Build history of the part. All positions in model axes, mm. Give positions to 0.01 mm unless a question says otherwise; leave off trailing zeros. Loops run counter-clockwise (first coordinate to the right, second up) from the corner with the lowest first, then second, coordinate; pieces in that order, holes last. Notation, with made-up numbers: (-39, 13) -> (12, 13) arc R17 cw to (12, 41) -> close; hole circle Ø2 at (-29.75, -23.75). An arc over 180 degrees is marked (long way). One line per question, with ' | ' between items. Start each with the question number.
(1) Slice it at B-B, the plane y = 7.5. Write the cut outline in (x, z).
(2) Mould opens along X. For faces 1 (the face through (2.37, 8.49, -2.08)), 2 (the face through (0, 8, -49)), 3 (the face through (3, 13, -1)) say: pulls with the +X half, pulls with the -X half, needs draft (parallel to the pull), parting line crosses it, or undercut.
(3) Slice it at A-A, the plane z = -6.4. Write the cut outline in (x, y), then the cut area to 3 significant figures.
(4) Slice it at C-C, the plane x = 2.5. Write the cut outline in (y, z).
(5) Flat gauge pins, fed straight in: pin 1 Ø1 at (x, y) = (0.5, 11.5) entering from +Z; pin 2 Ø1.5 at (x, y) = (4.5, 3.5) entering from -Z. Where does each tip first touch, or does it go through?
(6) Drill centre lines: L1, parallel to X at y = 7.5, z = -1.4; L2, parallel to Y at x = 2.75, z = -6.4; L3, parallel to Y at x = 2.5, z = -3. Where is each one in solid material? Low to high. Write a range as from..to.
```python
from build123d import *

# Parameters (mm, degrees)
SKETCH_1_W          = 100
SKETCH_1_H          = 15
EXTRUDE_1_DEPTH     = 5
SKETCH_2_R          = 2.4
CUT_EXTRUDE_1_DEPTH = 5
FILLET_1_R          = 5
SKETCH_4_R          = 1
CUT_EXTRUDE_2_DEPTH = 7


with BuildPart() as part:
    # 草图1 → 凸台-拉伸1 (new body)
    with BuildSketch(Plane(origin=(0, 0, 0), x_dir=(0, 0, -1), z_dir=(1, 0, 0))):
        with Locations((50, 7.5)):
            Rectangle(SKETCH_1_W, SKETCH_1_H)
    extrude(amount=EXTRUDE_1_DEPTH)

    # 草图2 → 切除-拉伸1 (cut)
    with BuildSketch(Plane(origin=(5, 0, 0), x_dir=(0, 0, -1), z_dir=(1, 0, 0))):
        with Locations((6.4, 7.5)):
            Circle(SKETCH_2_R)
    extrude(amount=-CUT_EXTRUDE_1_DEPTH, mode=Mode.SUBTRACT)

    # 圆角1
    fillet_1_edges = [part.edges().sort_by_distance(p)[0] for p in [
        (2.5, 15, 0),
        (2.5, 15, -100),
        (2.5, 0, -100),
        (2.5, 0, 0),
    ]]
    fillet(fillet_1_edges, radius=FILLET_1_R)

    # 草图4 → 切除-拉伸2 (cut)
    with BuildSketch(Plane.XY):
        with Locations((2.5, 7.5)):
            Circle(SKETCH_4_R)
    extrude(amount=-CUT_EXTRUDE_2_DEPTH, mode=Mode.SUBTRACT)


solid = part.part
```
Final values:
1) outline: (0, -100) -> (5, -100) -> (5, -8.8) -> (0, -8.8) -> close; (0, -4) -> (1.5, -4) -> (1.5, 0) -> (0, 0) -> close; (3.5, -4) -> (5, -4) -> (5, 0) -> (3.5, 0) -> close
2) face 1: undercut | face 2: pulls with the -X half | face 3: needs draft
3) outline: (0, 0) -> (5, 0) -> (5, 5.1) -> (0, 5.1) -> close; (0, 9.9) -> (5, 9.9) -> (5, 15) -> (0, 15) -> close | area: 51.0 mm2
4) outline: (0, -95) arc R5 ccw to (5, -100) -> (10, -100) arc R5 ccw to (15, -95) -> (15, -5) arc R5 ccw to (10, 0) -> (8.5, 0) -> (8.5, -4.22) arc R2.4 cw (long way) to (6.5, -4.22) -> (6.5, 0) -> (5, 0) arc R5 ccw to (0, -5) -> close
5) pin 1: z = -0.1 | pin 2: z = -99.94
6) L1: 0..1.5, 3.5..5 | L2: 0..5.1, 9.9..15 | L3: 0.42..6.5, 8.5..14.58
